Source: CAD feature listing. Evaluate the final solid. Frame: model axes, mm. A direction names the side the tool comes from. Give positions to 0.01 mm unless a question says otherwise; leave off trailing zeros. Order: outer loops, then holes, each group sorted by start corner. A loop starts at its lowest first (then second) coordinate and runs counter-clockwise, first axis right, second up. Notation, with made-up numbers: M -14,32 L 3,32 A5 cw 3,38 Z; hole C 14,6 d7. An arc over 180 degrees is marked long. Return JSON: item names as keys, results as strings.
Autodesk Fusion 360 part; units mm, degrees
sketch "Sketch1" plane through (0, 0, 0) normal (0, 0, 1) x (1, 0, 0) in component "LM6LUU"
  circle A0 centre (0, 0) radius 6
  circle A1 centre (0, 0) radius 3
  dimension "d1" = 12
  dimension "d2" = 6
extrude "Extrude1" add sketch "Sketch1" along normal blind 34 makes body 1 in component "LM6LUU"
copy_body "CutPasteBodies1" bodies 1 removing the originals makes body 2 in component "LM6LUU"
component "LM6LUU" placed x (1, 0, 0) y (0, 1, 0) z (0, 0, 1) at (0, 0, 0)

Autodesk Fusion 360 part; units mm, degrees
sketch "Back" plane through (0, 0, 0) normal (0, 0, 1) x (1, 0, 0) in component "X Carriage"
  line L0 (17.75, 23.5) -> (-17.75, 23.5) construction
  line L1 (-17.75, 23.5) -> (-17.75, -23.5)
  line L2 (-17.75, -23.5) -> (17.75, -23.5)
  line L3 (17.75, -23.5) -> (17.75, 23.5)
  line L4 (0, 23.5) -> (0, -23.5) construction
  line L5 (-17.75, 23.5) -> (-17.75, 27.7)
  line L6 (-17.75, 27.7) -> (-15.1, 27.7)
  line L7 (17.75, 23.5) -> (17.75, 30.5)
  line L8 (17.75, 30.5) -> (15.1, 30.5)
  line L9 (15.1, 30.5) -> (15.1, 23.5)
  line L10 (-15.1, 27.7) -> (-15.1, 23.5)
  line L11 (-15.1, 23.5) -> (15.1, 23.5)
  line L12 (-15.1, 21) -> (15.1, 21)
  line L13 (15.1, 21) -> (15.1, -6.5)
  line L14 (15.1, -6.5) -> (-15.1, -6.5)
  line L15 (-15.1, -6.5) -> (-15.1, 21)
  line L16 (-15.1, -9) -> (15.1, -9)
  line L17 (15.1, -9) -> (15.1, -23.5)
  line L18 (-15.1, -9) -> (-15.1, -23.5)
  line L19 (15.1, -21) -> (-15.1, -21)
  line L20 (-9.75, 0) -> (9.75, 0) construction
  circle A0 centre (-9.75, 0) radius 1.6
  circle A1 centre (9.75, 0) radius 1.6
  circle A2 centre (-9.75, 0) radius 3.5
  circle A3 centre (9.75, 0) radius 3.5
  line L21 (15.1, -7.75) -> (-15.1, -7.75)
  line L22 (-15.1, -7.75) -> (-15.1, -6.5)
  line L23 (15.1, -7.75) -> (15.1, -6.5)
  line L24 (17.75, 9.2) -> (19.75, 9.2)
  line L25 (19.75, 9.2) -> (19.75, 5.3)
  line L26 (19.75, 5.3) -> (17.75, 5.3)
  line L27 (-17.75, 9.2) -> (-19.75, 9.2)
  line L28 (-19.75, 9.2) -> (-19.75, 5.3)
  line L29 (-19.75, 5.3) -> (-17.75, 5.3)
  line L30 (-4.5, -2.7) -> (4.5, -2.7)
  line L31 (4.5, -2.7) -> (4.5, 6.3)
  line L32 (4.5, 6.3) -> (-4.5, 6.3)
  line L33 (-4.5, 6.3) -> (-4.5, -2.7)
  line L34 (-3, -2.7) -> (-3, 3.3)
  line L35 (-3, 3.3) -> (3, 3.3)
  line L36 (3, 3.3) -> (3, -2.7)
  circle A4 centre (9.75, 0) radius 2.7
  circle A5 centre (-9.75, 0) radius 2.7
  line L37 (-15.1, 21) -> (-15.1, 23.5)
  line L38 (15.1, 21) -> (15.1, 23.5)
  line L39 (-15.1, 9) -> (15.1, 9)
  point P0 (0, 21)
  point P1 (0, -2.7)
  point P2 (0, 3.3)
  dimension "d1" = 35.5
  dimension "d2" = 47
  dimension "d3" = 4.2
  dimension "d5" = 7
  dimension "d7" = 30.2
  dimension "d8" = 27.5
  dimension "d9" = 2.5
  dimension "d10" = 2.5
  dimension "d11" = 2.5
  dimension "d12" = 19.5
  dimension "d13" = 3.2
  dimension "d14" = 3.2
  dimension "d15" = 7
  dimension "d16" = 7
  dimension "d17" = 21
  dimension "d18" = 1.25
  dimension "d20" = 3.9
  dimension "d21" = 2
  dimension "d22" = 28.8
  dimension "d23" = 9
  dimension "d24" = 9
  dimension "d25" = 6
  dimension "d26" = 6
  dimension "d27" = 5.4
  dimension "d28" = 5.4
  dimension "d37" = 12
extrude "Extrude1" add sketch "Back" along normal blind 21.25 contours L1 L2 L3 L5 L6 L7 L8 L9 L10 L13 L15 L16 L17 L18 L21 L22 L23 L37 L38 makes body 1 in component "X Carriage"
extrude "Extrude2" add sketch "Back" along normal blind 19.25 contours L11 L12 L37 L38 | L14 L21 L22 L23 | A2 | A3 | A4 | A5 bodies 1 makes body 2 at (13.2326, -0.3485, 12.8333) makes body 3 at (-6.2674, -0.3485, 12.8333) in component "X Carriage"
extrude "Extrude3" add sketch "Back" along normal blind 8.5 contours L2 L17 L18 L19 bodies 1 in component "X Carriage"
extrude "Extrude4" add sketch "Back" along normal blind 8.45 contours L13 L14 L15 L39 | L30 L34 L35 L36 bodies 1 2 3 in component "X Carriage"
sketch "Side" plane through (17.75, 0, 0) normal (1, 0, 0) x (0, 1, 0) in component "X Carriage"
  line L0 (-23.5, 0) -> (30.5, 0) construction
  line L1 (30.5, 21.25) -> (-23.5, 21.25) construction
  line L2 (-23.5, 21.25) -> (-23.5, 0) construction
  circle A0 centre (15, 0) radius 6
  circle A1 centre (-15, 0) radius 6
  circle A2 centre (-15, 0) radius 8.5
  circle A3 centre (15, 0) radius 8.5
  line L3 (23.5, 0) -> (23.5, 19.25) construction
  line L4 (9, 8.45) -> (-6.5, 8.45) construction
  line L5 (9, 0) -> (9, 8.45) construction
  line L6 (-9, 0) -> (-9, 21.25) construction
  line L7 (-6.5, 8.45) -> (-6.5, 19.25) construction
  line L8 (-6.5, 0) -> (-6.5, 3.8)
  line L9 (6.5, 0) -> (6.5, 3.8)
  line L10 (-6.5, 3.8) -> (6.5, 3.8)
  line L11 (-6.5, 0) -> (6.5, 0)
  line L12 (-2.7, 3.8) -> (-2.7, 5.25)
  line L13 (-2.7, 5.25) -> (2.7, 5.25)
  line L14 (2.7, 5.25) -> (2.7, 3.8)
  line L15 (0, 5.25) -> (0, 3.8) construction
  line L16 (-23.5, 0) -> (23.5, 0)
  line L17 (30.5, 21.25) -> (30.5, 16.1)
  line L18 (28.5, 14.1) -> (23.5, 14.1) construction
  line L19 (25, 15.1) -> (27.5, 15.1)
  line L20 (23.5, 14.1) -> (25, 14.1)
  line L21 (25, 14.1) -> (25, 15.1)
  line L22 (27.5, 15.1) -> (27.5, 14.1)
  line L23 (30.5, 14.1) -> (27.5, 14.1) construction
  arc A4 (28.5, 14.1) -> (30.5, 16.1) centre (28.5, 16.1) ccw
  line L24 (30.5, 16.1) -> (30.5, 0)
  line L25 (30.5, 0) -> (23.5, 0)
  line L26 (23.5, 0) -> (23.5, 14.1)
  line L27 (28.5, 14.1) -> (27.5, 14.1)
  line L28 (30.5, 0) -> (30.5, 21.25)
  dimension "d38" = 12
  dimension "d39" = 12
  dimension "d40" = 17
  dimension "d41" = 17
  dimension "d42" = 30
  dimension "d43" = 3.8
  dimension "d44" = 3.8
  dimension "d45" = 1.45
  dimension "d46" = 13
  dimension "d47" = 5.4
  dimension "d48" = 7.15
  dimension "d49" = 2.5
  dimension "d50" = 1.5
  dimension "d51" = 1
  dimension "d52" = 7
  dimension "d53" = 2
extrude "Extrude5" cut sketch "Side" against normal blind 35.5 contours A0 L16 | A0 L16 | L8 L9 L10 L11 L16 | A1 L16 | A1 L16 bodies 1 in component "X Carriage"
extrude "Extrude6" add sketch "Side" along normal blind -33 and the other way blind 2.5 contours A0 A3 L16 | A1 A2 L16 picked at (22.635, -0.4223) picked at (-7.3873, -0.7204) bodies 1 in component "X Carriage"
extrude "Extrude7" cut sketch "Side" against normal blind 2.65 contours L19 L20 L21 L22 A4 L24 L25 L26 L27 L28 bodies 1 in component "X Carriage"
fillet "Fillet1" radius 2 1 edges at (-16.425, 27.7, 0) on bodies 1 in component "X Carriage"
fillet "Fillet2" radius 8 3 edges at (16.425, -23.5, 21.25) (-16.425, -23.5, 21.25) (16.425, -23.5, 21.25) on bodies 1 in component "X Carriage"
extrude "Extrude8" cut sketch "Side" against normal blind 14 contours L10 L12 L13 L14 bodies 1 in component "X Carriage"
extrude "Extrude9" cut sketch "Side" along normal blind 14 from surface at -35.5 contours L10 L12 L13 L14 bodies 1 in component "X Carriage"
extrude "Extrude10" cut sketch "Back" along normal blind 3 from surface at 5.25 contours A4 | A5 bodies 1 in component "X Carriage"
sketch "Belt Catch" plane through (0, 3.3, 0) normal (0, 1, 0) x (-1, 0, 0) in component "X Carriage"
  line L0 (-3, 3.8) -> (3, 3.8)
  line L1 (3, 3.8) -> (3, 8.45)
  line L2 (3, 8.45) -> (-3, 8.45)
  line L3 (-3, 8.45) -> (-3, 3.8)
  line L4 (-3, 8.45) -> (3, 8.45)
  line L5 (-3, 3.8) -> (-3, 8.45)
  line L6 (3, 3.8) -> (3, 8.45)
  line L7 (-3, 3.8) -> (3, 3.8)
  line L8 (-3, 6.45) -> (3, 6.45)
  line L9 (0, 6.45) -> (0, 8.45) construction
  line L10 (-0.375, 6.45) -> (-0.375, 7.075)
  line L11 (-0.375, 7.075) -> (0.375, 7.075) construction
  line L12 (0.375, 7.075) -> (0.375, 6.45)
  arc A0 (0.375, 7.075) -> (-0.375, 7.075) centre (0, 7.075) ccw
  line L13 (-1.625, 7.075) -> (-1.625, 6.45)
  arc A1 (-1.625, 7.075) -> (-2.375, 7.075) centre (-2, 7.075) ccw
  line L14 (-2.375, 6.45) -> (-2.375, 7.075)
  line L15 (2.375, 7.075) -> (2.375, 6.45)
  arc A2 (2.375, 7.075) -> (1.625, 7.075) centre (2, 7.075) ccw
  line L16 (1.625, 6.45) -> (1.625, 7.075)
  point P0 (0, 7.075)
  dimension "d72" = 2
  dimension "d73" = 0.625
  dimension "d74" = 0.75
  dimension "d77" = 2
  dimension "d78" = 0
extrude "Extrude11" cut sketch "Belt Catch" against normal blind 6 contours L1 L2 L3 L4 L5 L6 L8 L10 L12 A0 L13 A1 L14 L15 A2 L16 bodies 1 in component "X Carriage"
sketch "Sping Catch" plane through (-17.75, 0, 0) normal (-1, 0, 0) x (0, -1, 0) in component "X Carriage"
  line L0 (-2.7, 3.8) -> (-2.7, 5.25)
  line L1 (-2.7, 5.25) -> (2.7, 5.25)
  line L2 (2.7, 5.25) -> (2.7, 3.8)
  line L3 (2.7, 3.8) -> (6.5, 3.8)
  line L4 (6.5, 3.8) -> (6.5, 0)
  line L5 (6.5, 0) -> (9, 0)
  arc A0 (21, 0) -> (9, 0) centre (15, 0) ccw
  line L6 (21, 0) -> (23.5, 0)
  line L7 (23.5, 0) -> (23.5, 13.25)
  arc A1 (23.5, 13.25) -> (15.5, 21.25) centre (15.5, 13.25) ccw
  line L8 (15.5, 21.25) -> (-27.7, 21.25)
  line L9 (-27.7, 21.25) -> (-27.7, 2)
  arc A2 (-27.7, 2) -> (-25.7, 0) centre (-25.7, 2) ccw
  line L10 (-25.7, 0) -> (-21, 0)
  arc A3 (-9, 0) -> (-21, 0) centre (-15, 0) ccw
  line L11 (-9, 0) -> (-6.5, 0)
  line L12 (-6.5, 0) -> (-6.5, 3.8)
  line L13 (-6.5, 3.8) -> (-2.7, 3.8)
  line L14 (-27.7, 2) -> (-27.7, 21.25)
  line L15 (-27.7, 21.25) -> (15.5, 21.25)
  line L16 (-9.2, 21.25) -> (-8.85, 16.45)
  line L17 (-8.85, 16.45) -> (-5.65, 16.45)
  line L18 (-5.65, 16.45) -> (-5.3, 21.25)
  line L19 (-9.2, 21.25) -> (-5.3, 21.25)
  line L20 (-7.25, 21.25) -> (-7.25, 16.45) construction
  arc A4 (-8.85, 16.45) -> (-5.65, 16.45) centre (-7.25, 16.5667) ccw
  line L21 (-5.3, 0) -> (-5.3, 21.25) construction
  line L22 (-9.2, 0) -> (-9.2, 21.25) construction
  arc A5 (-8.9229, 17.45) -> (-5.5771, 17.45) centre (-7.25, 18.3493) ccw
  point P0 (-9.2, 0)
  point P1 (-5.3, 0)
  dimension "d82" = 3.2
  dimension "d83" = 4.8
  dimension "d84" = 1.6026
  dimension "d91" = 3.9
  dimension "d92" = 1
extrude "Extrude12" add sketch "Sping Catch" along normal blind 2.1 contours L8 L15 L16 L18 L19 A5 | L16 L17 A5 | L17 L18 A5 | L17 A4 bodies 1 in component "X Carriage"
extrude "Extrude13" cut sketch "Sping Catch" along normal blind 1.1 contours L17 A4 bodies 1 in component "X Carriage"
mirror "Mirror1" about plane through (0, 0, 0) normal (1, 0, 0) of "Extrude12", "Extrude13" in component "X Carriage"
component "X Carriage" placed x (1, 0, 0) y (0, 1, 0) z (0, 0, 1) at (0, 0, 0)
equation "d31 = 21.25 mm - 2 mm"
equation "d35 = 21.25 mm - 12.8 mm"
equation "d56 = -35.50 mm + 2.5 mm"
equation "d73 = 1 mm - ( 0.75 / 2 ) * 1 mm"
1. Ray query, probe 1 along Y at (x, z) = (9.75, 6.35); probe 2 along Y at (x, z) = (9.75, 17.25); probe 3 along Y at (x, z) = (0, 16.75). Return the intervals inside material, ascending.
Evaluation:
{"probe 1": "y = -23.5 to -21, -9 to -2.7, 2.7 to 9, 21 to 23.5", "probe 2": "y = -9 to -6.5, -3.5 to -1.6, 1.6 to 3.5, 21 to 23.5", "probe 3": "y = -9 to -6.5, 21 to 23.5"}
2. Section query A-A (y = 19). Return loops of the section in (x, z), then the cut area to 3 significant figures.
Evaluation:
{"outline": "M -17.75,4.47 L -15.1,4.47 L -15.1,21.25 L -17.75,21.25 Z; M -15.25,-7.5 L 15.25,-7.5 L 15.25,-4.47 L -15.25,-4.47 Z; M 15.1,4.47 L 17.75,4.47 L 17.75,21.25 L 15.1,21.25 Z", "area": "181 mm^2"}
3. Draft query along Y for faces 1 (the face through (15.25, -15, -7)), 2 (the face through (18.785, 9.023, 18.816)), 3 (the face through (0.213, -15.187, -8.498)). Return one class per face: pulls with the +Y half, pulls with the -Y half, needs draft (parallel to the pull), parting line crosses it, or undercut.
Evaluation:
{"face 1": "needs draft", "face 2": "pulls with the +Y half", "face 3": "undercut"}
4. Set-up query: faces 4 (the face through (0, -22, 8.5)), 5 (the face through (15.25, 15, -7)), 6 (the face through (16, 24, 14.1)), 7 (the face through (-11, 2.7, 5)). Return all of +Z, -Z, +X, -X, +Y, -Y with unobstructed straight access to the full face (end or side cutting, diameter ignored); none if empty.
Evaluation:
{"face 4": "+Z, -Y", "face 5": "-Z, +X, +Y, -Y", "face 6": "-Z, +X, +Y", "face 7": "-Z, -X"}
5. Section query B-B (y = 0). State how many separate pieces and enclosed holes the cut face has, then the cut area to 3 significant figures.
Evaluation:
{"separate pieces": "5", "enclosed holes": "0", "area": "219 mm^2"}
6. First-contact query: pin 1 (6 mm diameter, centred on x = 2, y = 24.5, fed in from +Z); pin 2 (5 mm diameter, centred on x = 8.5, y = 23.5, fed in from -Z); pin 3 (12 mm diameter, centred on x = 8.5, z = 10, fed in from -Y); pin 4 (2 mm diameter, centred on y = 20, z = 15.5, fed in from +X). Flat tips, straight axial feed; report the tip coordinate or a pass-through.
Evaluation:
{"pin 1": "stops at z = 19.25", "pin 2": "stops at z = -6.02", "pin 3": "stops at y = -23.5", "pin 4": "stops at x = 17.75"}
